Design review of the part shown in the three views and the two pictorial views. Dimensions are in mm from the part's minimum x, y and z. Round coordinates to 2 decimals unless told otherwise and drop trailing zeros. Write each loop counter-clockwise with the first axis right and the second up, starting at its lowest first coordinate (ties: lowest second). Pieces come first, ordered by that corner, then holes. Notation, with made-up numbers: (-15, 69) -> (12, 69) arc R13 ccw to (12, 89) -> close; hole circle Ø3 at (36.5, -19.5). An arc over 180 degrees is marked (long way). One line per question, with ' | ' between items. Start each with the question number.
1) For probe 1 along Z at (x, y) = (19, 26.5); probe 2 along Y at (x, z) = (93.5, 72.5); probe 3 along X at (y, z) = (18.75, 149.5), list the stretches that pass through material, from the lowest coordinate up.
2) Consider section A-A (z = 155). Give the boundary of the cut face in (x, y), then the cut area to 3 significant figures.
3) Consider section C-C (x = 261.5). Give the boundary of the cut face in (y, z).
4) Consider section D-D (z = 134). Give the boundary of the cut face in (x, y).
5) Insertion check: pin 1 Ø2 at (x, y) = (15, 26.5) entering from +Z; pin 2 Ø1 at (y, z) = (16.5, 157.5) entering from +X; pin 3 Ø2 at (x, z) = (177, 68.5) entering from +Y. Each pin has a flat end and moves straight along its axis. Give the tip position at first contact, or say it passes through.
6) Mouldability with a two-part tool opening along X and no side actions: class the marked faces 1 and 2 as +X half, -X half, draft (parallel to the pull), parting line (faces both ways), or undercut.
7) Consider section B-B (y = 13). Give the boundary of the cut face in (x, z), then the cut area to 3 significant figures.
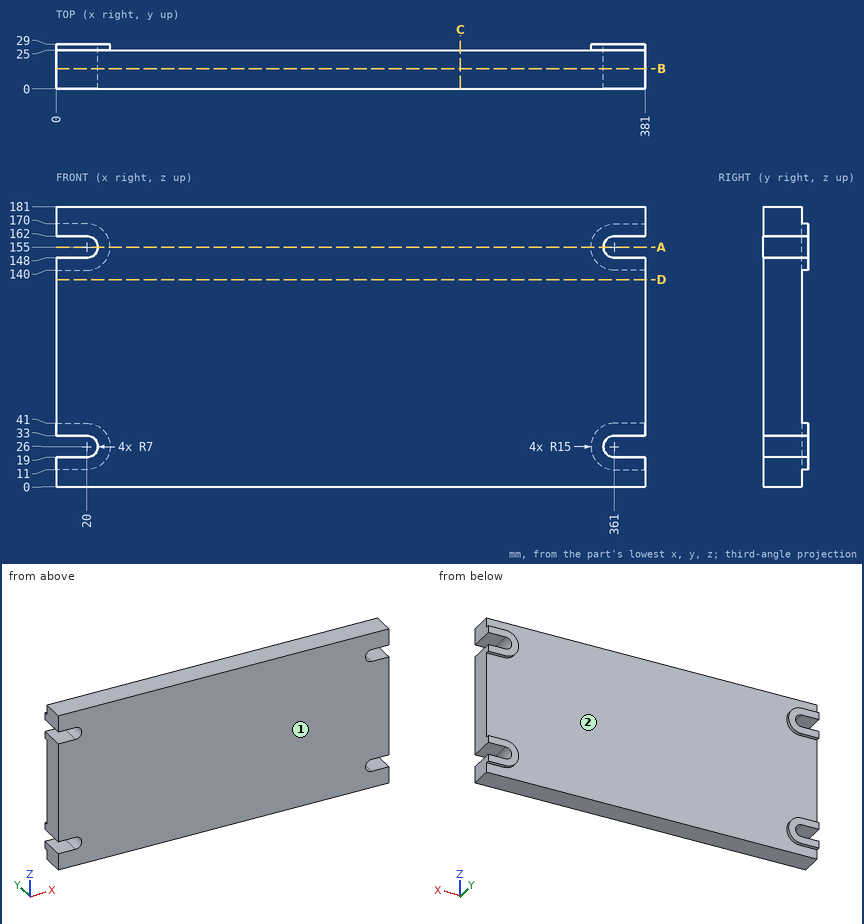
From the geometry:
1) probe 1: z = 11 to 19, 33 to 41, 140 to 148, 162 to 170 | probe 2: y = 0 to 25 | probe 3: x = 24.33 to 356.67
2) outline: (27, 0) -> (354, 0) -> (354, 29) -> (346, 29) -> (346, 25) -> (35, 25) -> (35, 29) -> (27, 29) -> close | area: 8,240 mm2
3) outline: (0, 0) -> (25, 0) -> (25, 181) -> (0, 181) -> close
4) outline: (0, 0) -> (381, 0) -> (381, 25) -> (0, 25) -> close
5) pin 1: stops at z = 170 | pin 2: stops at x = 354.68 | pin 3: stops at y = 25
6) face 1: draft | face 2: undercut
7) outline: (0, 0) -> (381, 0) -> (381, 19) -> (361, 19) arc R7 cw to (361, 33) -> (381, 33) -> (381, 148) -> (361, 148) arc R7 cw to (361, 162) -> (381, 162) -> (381, 181) -> (0, 181) -> (0, 162) -> (20, 162) arc R7 cw to (20, 148) -> (0, 148) -> (0, 33) -> (20, 33) arc R7 cw to (20, 19) -> (0, 19) -> close | area: 67,500 mm2
